from build123d import *

# Parameters (mm, degrees)
PAD_DEPTH       = 10
SKETCH002_R     = 11
POCKET_DEPTH    = 7
SKETCH003_R     = 5.9
POCKET001_DEPTH = 5
SKETCH004_R     = 2.6
POCKET002_DEPTH = 5


with BuildPart() as part:
    # Sketch → Pad (new body)
    with BuildSketch(Plane.XZ):
        with BuildLine():
            Line((-14, 15), (-14, 0))
            ThreePointArc((-14, 0), (0, -14), (14, 0))
            Line((14, 0), (14, 15))
            Line((14, 15), (-14, 15))
        make_face()
    extrude(amount=PAD_DEPTH)

    # Sketch002 (on Face5 of Pad) → Pocket (cut)
    with BuildSketch(Plane(origin=(0, 0, 0), x_dir=(1, 0, 0), z_dir=(0, 1, 0))):
        Circle(SKETCH002_R)
    extrude(amount=-POCKET_DEPTH, mode=Mode.SUBTRACT)

    # Sketch003 (on Face5 of Pocket) → Pocket001 (cut)
    with BuildSketch(Plane.XZ.offset(10)):
        Circle(SKETCH003_R)
    extrude(amount=-POCKET001_DEPTH, mode=Mode.SUBTRACT)

    # Sketch004 (on Face5 of Pocket001) → Pocket002 (cut)
    with BuildSketch(Plane.XZ.offset(10)):
        with Locations((0, 6.2)):
            Circle(SKETCH004_R)
    extrude(amount=-POCKET002_DEPTH, mode=Mode.SUBTRACT)


solid = part.part
Geometry check sheet. Reference: the model listing, model coordinates, mm. Round coordinates to 2 decimals unless told otherwise and drop trailing zeros. Order: outer loops, then holes, each group sorted by start corner. A loop starts at its lowest first (then second) coordinate and runs counter-clockwise, first axis right, second up. Notation, with made-up numbers: M -11.5,52 L -4.5,52 A36 ccw -4.5,90 Z; hole C 53,43.5 d6. An arc over 180 degrees is marked long. Write each question's results on one line, items separated by ' | '. Start each with the question number.
1. Cross-section at D-D on x = 12.25. Record the boundary of the cut face in (y, z), plus the area to 3 significant figures.
2. Cross-section at C-C on y = -5.75. Record the boundary of the cut face in (x, z).
3. Material ranges on L1, parallel to X at y = -8.2, z = 6.2; L2, parallel to Z at x = 0, y = -7.65; L3, parallel to Z at x = 0, y = -2.25, recorded low to high. Write a range as from..to.
4. Draft check along X on faces 1 (the face through (-14, -5, 8)), 2 (the face through (5, -7, 5)), 3 (the face through (-2.38, -3.45, 10.74)), 4 (the face through (0, -5, -14)). Enter one of: pulls with the +X half, pulls with the -X half, needs draft (parallel to the pull), parting line crosses it, or undercut.
5. Go/stop test with flat-tipped pins: P1, Ø5, axis at y = -9, z = -10.5, coming from the -X side; P2, Ø2, axis at y = -8.5, z = -9, coming from the +X side. Record where each tip stops, or that it passes through.
6. Cross-section at B-B on z = -5. Record the boundary of the cut face in (x, y), plus the area to 3 significant figures.
7. Cross-section at A-A on x = 0. Record the boundary of the cut face in (y, z), plus the area to 3 significant figures.
Resolved:
1) outline: M -10,-6.78 L 0,-6.78 L 0,15 L -10,15 Z | area: 218 mm2
2) outline: M -14,0 A14 ccw 14,0 L 14,15 L -14,15 Z; hole C 0,0 d22
3) L1: -14..-2.6, 2.6..14 | L2: -14..-5.9, 8.8..15 | L3: -14..-11, 11..15
4) face 1: pulls with the -X half | face 2: undercut | face 3: undercut | face 4: parting line crosses it
5) P1: x = -11.49 | P2: x = 11.49
6) outline: M -13.08,-10 L -3.13,-10 L -3.13,-7 L -9.8,-7 L -9.8,0 L -13.08,0 Z; M 3.13,-10 L 13.08,-10 L 13.08,0 L 9.8,0 L 9.8,-7 L 3.13,-7 Z | area: 106 mm2
7) outline: M -10,-14 L 0,-14 L 0,-11 L -7,-11 L -7,-5.9 L -10,-5.9 Z; M -10,8.8 L -7,8.8 L -7,11 L 0,11 L 0,15 L -10,15 Z | area: 91.9 mm2
